Autodesk Inventor part; units mm, degrees
ref_plane "YZ Plane" through (0, 0, 0) normal (1, 0, 0) x (0, 1, 0)
ref_plane "XZ Plane" through (0, 0, 0) normal (0, 1, 0) x (-1, 0, 0)
ref_plane "XY Plane" through (0, 0, 0) normal (0, 0, 1) x (1, 0, 0)
sketch "Sketch1" plane through (0, 0, 0) normal (0, 0, 1) x (1, 0, 0)
  line L0 (3.6662, 6.35) -> (7.3323, 0)
  line L1 (7.3323, 0) -> (3.6662, -6.35)
  line L2 (3.6662, -6.35) -> (-3.6662, -6.35)
  line L3 (-3.6662, -6.35) -> (-7.3323, 0)
  line L4 (-7.3323, 0) -> (-3.6662, 6.35)
  line L5 (-3.6662, 6.35) -> (3.6662, 6.35)
  circle A0 centre (0, 0) radius 12.7
  circle A1 centre (0, 0) radius 7.3323 construction
  dimension "d0" = 12.7
  dimension "d2" = 25.4
  dimension "d3" = 5.3677
extrude "Extrusion1" add sketch "Sketch1" against normal blind 6.35
properties part number "1_2x1-hexBearing" material "PC/ABS Plastic"
Check sheet for the modelled part. Datum: model origin and axes. Units: mm. A direction names the side the tool comes from. Round coordinates to 2 decimals unless told otherwise and drop trailing zeros. Order: outer loops, then holes, each group sorted by start corner. A loop starts at its lowest first (then second) coordinate and runs counter-clockwise, first axis right, second up. Notation, with made-up numbers: (-26.75, 12.5) -> (-4.75, 12.5) arc R29 ccw to (-4.75, 40.5) -> close; hole circle Ø6 at (-16, 19.5). An arc over 180 degrees is marked (long way). One line per item, written item: value. Start each with the question number.
Q1. Thickness scan on line 1 (Y direction, x = -0.25, z = -2); line 2 (Y direction, x = 6.25, z = -1); line 3 (X direction, y = 1.5, z = -2.25). Record the ranges inside material, lowest first.
Q2. Cross-section at D-D (y = 8). Record the boundary of the cut face in (x, z).
Q3. Cross-section at A-A (y = -6). Record the boundary of the cut face in (x, z).
Q4. Cross-section at B-B (x = 0). Record the boundary of the cut face in (y, z).
Q5. Set-up check for faces 1 (the face through (0, 6.35, -3)), 2 (the face through (-6, -3, 0)): record each of +Z, -Z, +X, -X, +Y, -Y from which the full face is reachable in a straight line by a thin tool's end or side.
Q6. Cross-section at C-C (z = -3.25). Record the boundary of the cut face in (x, y), and give its area (3 significant figures).
Q7. Gauge pin test, flat ends, axial feed: pin 1 Ø8 at (x, y) = (9, -8) entering from +Z; pin 2 Ø1.5 at (x, z) = (4.5, -1.5) entering from +Y; pin 3 Ø1 at (x, z) = (8.5, -4) entering from -Y. Record the tip position at first contact, or that the pin passes through.
Q8. Mould release check, pull along X, two halves, no side actions. Record for faces 3 (the face through (-6, -3, -6.35)), 4 (the face through (-2.75, -12.4, -3.13)), 5 (the face through (0, -6.35, -3)): pulls with the +X half, pulls with the -X half, needs draft (parallel to the pull), parting line crosses it, or undercut.
Completed:
1. line 1: y = -12.7 to -6.35, 6.35 to 12.7
1. line 2: y = -11.06 to -1.87, 1.87 to 11.06
1. line 3: x = -12.61 to -6.47, 6.47 to 12.61
2. outline: (-9.86, -6.35) -> (9.86, -6.35) -> (9.86, 0) -> (-9.86, 0) -> close
3. outline: (-11.19, -6.35) -> (-3.87, -6.35) -> (-3.87, 0) -> (-11.19, 0) -> close; (3.87, -6.35) -> (11.19, -6.35) -> (11.19, 0) -> (3.87, 0) -> close
4. outline: (-12.7, -6.35) -> (-6.35, -6.35) -> (-6.35, 0) -> (-12.7, 0) -> close; (6.35, -6.35) -> (12.7, -6.35) -> (12.7, 0) -> (6.35, 0) -> close
5. face 1: +Z, -Z
5. face 2: +Z, +X, -X, +Y, -Y
6. outline: circle Ø25.4 at (0, 0); hole (-7.33, 0) -> (-3.67, -6.35) -> (3.67, -6.35) -> (7.33, 0) -> (3.67, 6.35) -> (-3.67, 6.35) -> close
6. area: 367 mm²
7. pin 1: stops at z = 0
7. pin 2: stops at y = 12.13
7. pin 3: stops at y = -9.86
8. face 3: needs draft
8. face 4: parting line crosses it
8. face 5: undercut
